from build123d import *

# Parameters (mm, degrees)
SKETCH1_R             = 3.7
SKETCH1_R_2           = 2.4
HUB_DEPTH             = 3.9
SKETCH2_R             = 3.1
RIM_CUT_DEPTH         = 0.8
BLADE_DEPTH           = 1.1
BLADE_CURVE_DEPTH     = 23.16190425
BODY_MOVE_COPY1_ANGLE = 15
CIRPATTERN1_COUNT     = 3


with BuildPart() as part:
    # Sketch1 → Hub (new, symmetric)
    with BuildSketch(Plane(origin=(0, 0, 0), x_dir=(1, 0, 0), z_dir=(0, 1, 0))):
        with Locations(Location((0, 0, 0), (0, 0, 270))):
            Circle(SKETCH1_R)
        with Locations(Location((0, 0, 0), (0, 0, 270))):
            Circle(SKETCH1_R_2, mode=Mode.SUBTRACT)
    extrude(amount=HUB_DEPTH, both=True)

    # Sketch2 → Rim Cut (cut)
    with BuildSketch(Plane(origin=(0, 3.9, 0), x_dir=(1, 0, 0), z_dir=(0, 1, 0))):
        with Locations(Location((0, 0, 0), (0, 0, 270))):
            Circle(SKETCH2_R)
    rim_cut = extrude(amount=-RIM_CUT_DEPTH, mode=Mode.SUBTRACT)

    # Mirror1: Rim Cut across plane
    add(rim_cut.mirror(Plane.ZX), mode=Mode.SUBTRACT)


with BuildPart() as body_2:
    # Sketch3 → Blade (new, symmetric)
    with BuildSketch(Plane(origin=(0, 0, 0), x_dir=(1, 0, 0), z_dir=(0, 1, 0))):
        with BuildLine():
            Line((-2, 3.7), (-3.35, 6.55))
            Line((-3.35, 6.55), (-2.625, 20.5))
            ThreePointArc((-2.625, 20.5), (0, 21.5), (2.625, 20.5))
            Line((2.625, 20.5), (3.35, 6.55))
            Line((3.35, 6.55), (2, 3.7))
            Line((2, 3.7), (1.526315789, 2.7))
            Line((1.526315789, 2.7), (-1.526315789, 2.7))
            Line((-1.526315789, 2.7), (-2, 3.7))
        make_face()
    extrude(amount=BLADE_DEPTH, both=True)

    # Sketch4 → Blade Curve (cut, through all)
    with BuildSketch(Plane.XY):
        with BuildLine():
            Line((3.35, 0.6), (3.35, 1.1))
            Line((3.35, 1.1), (0, 1.1))
            ThreePointArc((0, 1.1), (1.693553955, 0.974311501), (3.35, 0.6))
        make_face()
        with BuildLine():
            ThreePointArc((-3.35, 0.6), (-1.693553955, 0.974311501), (0, 1.1))
            Line((0, 1.1), (-3.35, 1.1))
            Line((-3.35, 1.1), (-3.35, 0.6))
        make_face()
        with BuildLine():
            ThreePointArc((0, -1.1), (-1.693553955, -0.974311501), (-3.35, -0.6))
            Line((-3.35, -0.6), (-3.35, -1.1))
            Line((-3.35, -1.1), (0, -1.1))
        make_face()
        with BuildLine():
            ThreePointArc((3.35, -0.6), (1.693553955, -0.974311501), (0, -1.1))
            Line((0, -1.1), (3.35, -1.1))
            Line((3.35, -1.1), (3.35, -0.6))
        make_face()
    extrude(amount=-BLADE_CURVE_DEPTH, mode=Mode.SUBTRACT)


with BuildPart() as body_2_1:
    # Body-Move_Copy1: moved
    add(body_2.part.rotate(Axis((0, 0, 0), (0, 0, 1)), BODY_MOVE_COPY1_ANGLE))


with BuildPart() as cirpattern1_1:
    # CirPattern1: pattern copy
    add(body_2_1.part.rotate(Axis((0, 0, 0), (0, 1, 0)), 1 * 360 / CIRPATTERN1_COUNT))


with BuildPart() as cirpattern1_2:
    # CirPattern1: pattern copy
    add(body_2_1.part.rotate(Axis((0, 0, 0), (0, 1, 0)), 2 * 360 / CIRPATTERN1_COUNT))


with BuildPart() as cirpattern1_1_1:
    add(cirpattern1_1.part)

    # Combine1: union part, body 2, CirPattern1_2
    add(part.part)
    add(body_2_1.part)
    add(cirpattern1_2.part)


solid = cirpattern1_1_1.part
Could you check a few things on this model? Use its own coordinates, in mm. A direction names the side the tool comes from. Give positions to 0.01 mm unless a question says otherwise; leave off trailing zeros. Order: outer loops, then holes, each group sorted by start corner. A loop starts at its lowest first (then second) coordinate and runs counter-clockwise, first axis right, second up. Notation, with made-up numbers: (-18.5, 83.5) -> (33.5, 83.5) arc R28 cw to (33.5, 109.5) -> close; hole circle Ø4 at (16.5, 70.25). An arc over 180 degrees is marked (long way). Answer in a Markdown table with one row per item. Add a question column.
Item 1: Please list where these lines run through material, in increasing order: probe 1 along Z at (x, y) = (0, -1.75); probe 2 along X at (y, z) = (3.3, 0).
Item 2: Imagine slicing it at B-B (y = -2.5). List the corners of the cut face in (x, z) for me, and give its area (3 significant figures).
Item 3: I'm going to push flat-ended pins straight in: P1, Ø3.5, axis at x = 0, z = 0, coming from the +Y side; P2, Ø1, axis at x = 10, y = -0.5, coming from the -Z side. Where does each tip first touch, or does it pass through?
Item 4: Imagine slicing it at C-C (z = -13). List the corners of the cut face in (x, y) for me (1 decimal), and give its area (3 significant figures).
Item 5: We'd pull the mould along X, two halves only. Please class faces 6 (the flat face through (-10.18, -0.76, 9.22)), 7 (the flat face through (13.08, -0.76, 4.21)), 8 (the cylindrical face through (0.931, 3.506, 2.957)), 9 (the flat face through (-13.2, 0.8, 4.3)): pulls with the +X half, pulls with the -X half, needs draft (parallel to the pull), parting line crosses it, or undercut.
Item 6: For faces 1 (the cylindrical face through (-3.612, 0.055, -0.802)), 2 (the flat face through (10.359, 0.783, 9.304)), 3 (the cylindrical face through (0.931, -3.506, 2.957)), 4 (the flat face through (-2.893, -0.764, -13.427)), 5 (the flat face through (-2, 3.1, 2)), which set-ups out of +Z, -Z, +X, -X, +Y, -Y let a thin tool reach every point of the face, with its end or its side?
Item 7: Imagine slicing it at A-A (z = -9.5). List the corners of the cut face in (x, y) for me (1 decimal).
Result:
| question | item | result |
|---|---|---|
| 1 | probe 1 | -3.7 to -2.4, 2.4 to 3.7 |
| 1 | probe 2 | -3.7 to -3.1, 3.1 to 3.7 |
| 2 | outline | circle Ø7.4 at (0, 0); hole circle Ø4.8 at (0, 0) |
| 2 | area | 24.9 mm2 |
| 3 | P1 | through |
| 3 | P2 | z = 1.76 |
| 4 | outline | (-3.1, -0.1) -> (-2.7, -1.5) arc R11.5 ccw to (3.1, 0.1) -> (2.7, 1.5) arc R11.5 ccw to start |
| 4 | area | 11.7 mm2 |
| 5 | face 6 | undercut |
| 5 | face 7 | pulls with the +X half |
| 5 | face 8 | undercut |
| 5 | face 9 | pulls with the -X half |
| 6 | face 1 | none |
| 6 | face 2 | +Z, +Y |
| 6 | face 3 | -Y |
| 6 | face 4 | -Z, -X, -Y |
| 6 | face 5 | +Y |
| 7 | outline | (-3.3, -0.2) -> (-2.9, -1.5) arc R11.5 ccw to (3.3, 0.2) -> (2.9, 1.5) arc R11.5 ccw to start |
